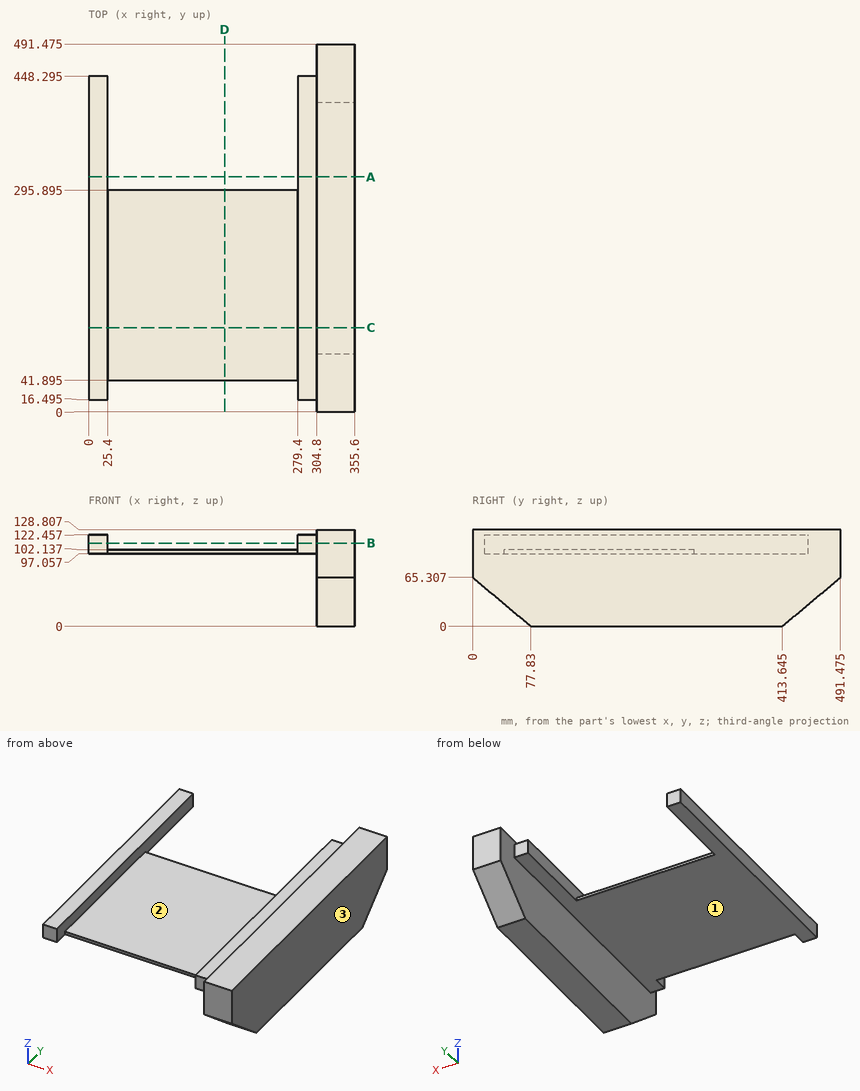
Source: three-view drawing plus pictorial views. Frame: mm from the lowest corner of the part. Round coordinates to 2 decimals unless told otherwise and drop trailing zeros. Loops run counter-clockwise (first coordinate to the right, second up) from the corner with the lowest first, then second, coordinate; pieces in that order, holes last. Notation, with made-up numbers: M 82,72 L 110,72 A12 ccw 110,88 Z; hole C -1.75,70.25 d9. An arc over 180 degrees is marked long. Put each result on its own line as item: value. Start each with the question number.
(1) Section query D-D (x = 182). Return loops of the section in (y, z) (1 decimal).
(2) Contact query for flat-ended pins moving along their axis: pin 1 Ø1.5 at (x, y) = (100, 161) entering from +Z; pin 2 Ø3 at (y, z) = (64.5, 67) entering from -X; pin 3 Ø7.5 at (x, z) = (9, 109) entering from +Y (1 decimal). Output: stop coordinate, or through.
(3) Material intervals for line 1 along X through (y, z) = (58, 112); line 2 along X through (y, z) = (468.5, 52.5); line 3 along Z through (x, y) = (205, 288), sorted ascending. Write a range as [from, to].
(4) Section query C-C (y = 112.5). Return loops of the section in (x, z), then the cut area to 3 significant figures.
(5) Section query A-A (y = 314). Return loops of the section in (x, z).
(6) Section query B-B (z = 111). Return loops of the section in (x, y) (1 decimal), then the cut area to 3 significant figures.
(7) Draft query along X for the marked faces 1, 2 and 3. Return one class per face: +X half, -X half, draft (parallel to the pull), parting line (faces both ways), or undercut.
Findings below:
1. outline: M 41.9,97.1 L 295.9,97.1 L 295.9,102.1 L 41.9,102.1 Z
2. pin 1: stops at z = 102.14
2. pin 2: stops at x = 304.8
2. pin 3: stops at y = 448.3
3. line 1: x = [0, 25.4], [279.4, 355.6]
3. line 2: x = [304.8, 355.6]
3. line 3: z = [97.06, 102.14]
4. outline: M 0,97.06 L 304.8,97.06 L 304.8,0 L 355.6,0 L 355.6,128.81 L 304.8,128.81 L 304.8,122.46 L 279.4,122.46 L 279.4,102.14 L 25.4,102.14 L 25.4,122.46 L 0,122.46 Z
4. area: 9,120 mm2
5. outline: M 0,97.06 L 25.4,97.06 L 25.4,122.46 L 0,122.46 Z; M 279.4,97.06 L 304.8,97.06 L 304.8,0 L 355.6,0 L 355.6,128.81 L 304.8,128.81 L 304.8,122.46 L 279.4,122.46 Z
6. outline: M 0,16.5 L 25.4,16.5 L 25.4,448.3 L 0,448.3 Z; M 279.4,16.5 L 304.8,16.5 L 304.8,0 L 355.6,0 L 355.6,491.5 L 304.8,491.5 L 304.8,448.3 L 279.4,448.3 Z
6. area: 46,900 mm2
7. face 1: draft
7. face 2: undercut
7. face 3: +X half
